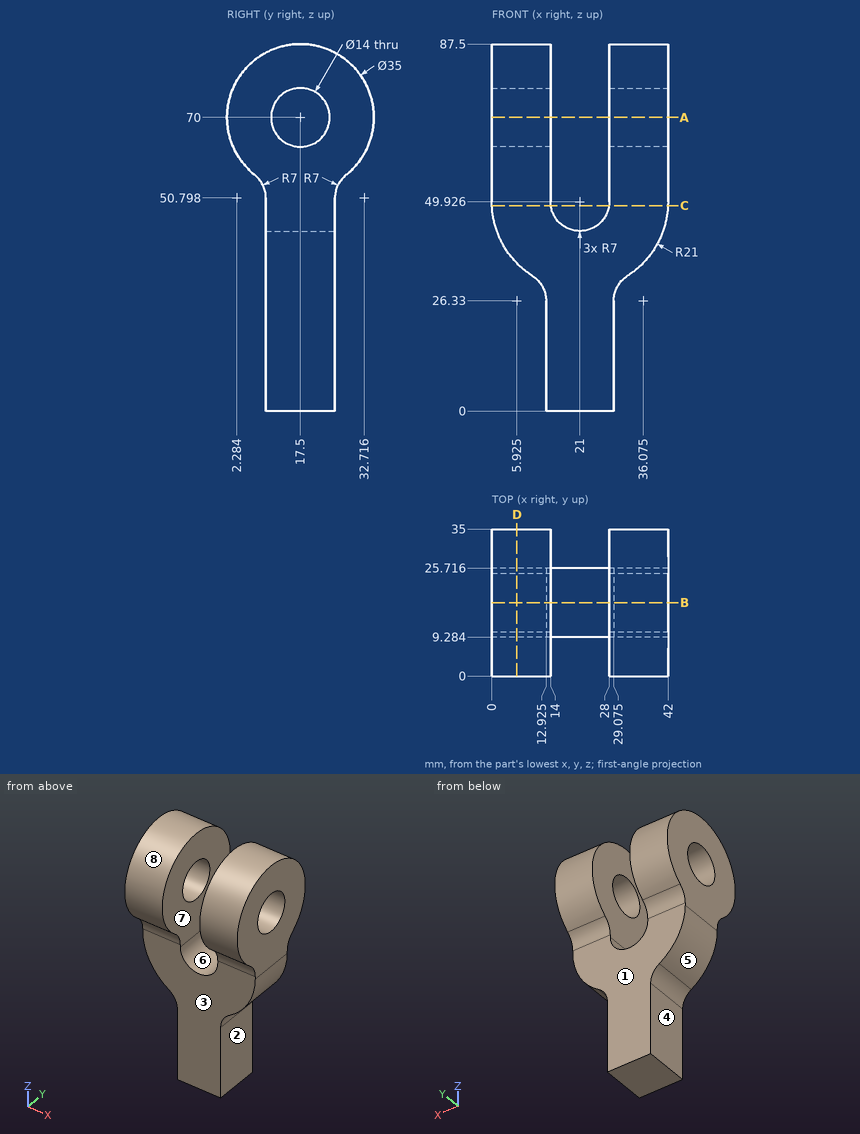
Answer from the drawing. Dimensions are ordinates in mm from the lowest x, y and z of the part. A direction names the side the tool comes from. Coordinates: 2 decimals unless noted, no trailing zeros. Write each loop counter-clockwise with the first axis right and the second up, starting at its lowest first coordinate (ties: lowest second). Pieces come first, ordered by that corner, then holes. Notation, with made-up numbers: M 81.25,8 L 97.25,8 A18 cw 97.25,35 Z; hole C 47.5,-22.5 d1. An arc over 180 degrees is marked long. Write item = value, one per line.
1. The part is cut by section D-D (x = 6). Determine the outline of the cut face in (y, z) (1 decimal), then the cut area to 3 significant figures.
Solution:
outline = M 6.6,56.3 A7 cw 9.3,50.8 L 9.3,35.2 L 25.7,35.2 L 25.7,50.8 A7 cw 28.4,56.3 A17.5 ccw long Z; hole C 17.5,70 d14
area = 1,110 mm2
2. Flat-ended cylindrical pins translate along their axes: pin 1 (8 mm diameter, centred on x = 4.5, y = 20.5, fed in from -Z); pin 2 (4 mm diameter, centred on x = 26, z = 23, fed in from +Y); pin 3 (1 mm diameter, centred on x = 5.5, y = 14.5, fed in from +Z). Find the tip coordinate at first contact, or state that the pin passes through.
Solution:
pin_1 = 33.05
pin_2 = 25.72
pin_3 = 87.32
3. Straight lines are drawn through the part: line 1 (X direction, y = 23, z = 74.5); line 2 (Y direction, x = 8, z = 70); line 3 (X direction, y = 20, z = 16.5) (1 decimal). For each, find the intervals that lie inside material, in ascending order. Write a range as from..to.
Solution:
line_1 = 0..14, 28..42
line_2 = 0..10.5, 24.5..35
line_3 = 12.9..29.1
4. The part is cut by section A-A (z = 70). Determine the outline of the cut face in (x, y).
Solution:
outline = M 0,0 L 14,0 L 14,10.5 L 0,10.5 Z; M 0,24.5 L 14,24.5 L 14,35 L 0,35 Z; M 28,0 L 42,0 L 42,10.5 L 28,10.5 Z; M 28,24.5 L 42,24.5 L 42,35 L 28,35 Z
5. The part is cut by section C-C (z = 49). Determine the outline of the cut face in (x, y).
Solution:
outline = M 0.02,9.28 L 14.06,9.28 L 14.06,25.72 L 0.02,25.72 Z; M 27.94,9.28 L 41.98,9.28 L 41.98,25.72 L 27.94,25.72 Z
6. The part is cut by section B-B (y = 17.5). Determine the outline of the cut face in (x, z) (1 decimal).
Solution:
outline = M 0,49.9 A21 ccw 9.7,32.2 A7 cw 12.9,26.3 L 12.9,0 L 29.1,0 L 29.1,26.3 A7 cw 32.3,32.2 A21 ccw 42,49.9 L 42,63 L 28,63 L 28,49.9 A7 cw 14,49.9 L 14,63 L 0,63 Z; M 0,77 L 14,77 L 14,87.5 L 0,87.5 Z; M 28,77 L 42,77 L 42,87.5 L 28,87.5 Z
7. Determine the mould class of the marked faces 5, 6, 7 and 8 for opening direction X: released by +X, released by -X, zero draft, split by the parting line, or undercut.
Solution:
face_5 = released by -X
face_6 = undercut
face_7 = undercut
face_8 = zero draft
8. For the marked faces 1, 2, 3 and 4, determine the directions among +Z, -Z, +X, -X, +Y, -Y from which every point of the face is accessible in a straight line to the end or side of a thin tool.
Solution:
face_1 = -Z, +X, -X, +Y
face_2 = -Z, +X, +Y, -Y
face_3 = -Z, +X, -X, -Y
face_4 = -Z, -X, +Y, -Y
